from build123d import *

# Parameters (mm, degrees)
SKETCH1_W           = 152.4
SKETCH1_H           = 50.8
BOSS_EXTRUDE1_DEPTH = 6.35
SKETCH2_R           = 1.8288
CUT_EXTRUDE1_DEPTH  = 6.35
SKETCH5_W           = 8.89
SKETCH5_H           = 11.765011578
CUT_EXTRUDE2_DEPTH  = 161.769159045


with BuildPart() as part:
    # Sketch1 → Boss-Extrude1 (new body)
    with BuildSketch(Plane(origin=(0, 0, 0), x_dir=(1, 0, 0), z_dir=(0, 1, 0))):
        with Locations((-76.2, 25.4)):
            Rectangle(SKETCH1_W, SKETCH1_H)
    extrude(amount=BOSS_EXTRUDE1_DEPTH)

    # Sketch2 → Cut-Extrude1 (cut)
    with BuildSketch(Plane(origin=(0, 6.35, 0), x_dir=(1, 0, 0), z_dir=(0, 1, 0))):
        with Locations(Location((-149.225, 44.45, 0), (0, 0, 270))):
            Circle(SKETCH2_R)
        with Locations(Location((-149.225, 25.4, 0), (0, 0, 270))):
            Circle(SKETCH2_R)
        with Locations(Location((-149.225, 6.35, 0), (0, 0, 270))):
            Circle(SKETCH2_R)
        with Locations(Location((-3.175, 25.4, 0), (0, 0, 270))):
            Circle(SKETCH2_R)
        with Locations(Location((-3.175, 44.45, 0), (0, 0, 270))):
            Circle(SKETCH2_R)
        with Locations(Location((-3.175, 6.35, 0), (0, 0, 270))):
            Circle(SKETCH2_R)
    extrude(amount=-CUT_EXTRUDE1_DEPTH, mode=Mode.SUBTRACT)

    # Sketch5 → Cut-Extrude2 (cut, through all)
    with BuildSketch(Plane(origin=(0, 6.35, 0), x_dir=(1, 0, 0), z_dir=(0, 1, 0))):
        with Locations((-117.221, 44.917494211)):
            Rectangle(SKETCH5_W, SKETCH5_H)
    extrude(amount=-CUT_EXTRUDE2_DEPTH, mode=Mode.SUBTRACT)


solid = part.part
Could you check a few things on this model? Use its own coordinates, in mm. A direction names the side the tool comes from. Coordinates: 2 decimals unless noted, no trailing zeros. Order: outer loops, then holes, each group sorted by start corner. A loop starts at its lowest first (then second) coordinate and runs counter-clockwise, first axis right, second up.
Q1. Will these pins go through, and if not, where does the flat tip stop? pin 1 (3 mm diameter, centred on x = -3.175, z = -6.35, fed in from +Y); pin 2 (3 mm diameter, centred on x = -118.5, y = 4.5, fed in from -Z) (3 decimals).
Q2. Which directions (+Z, -Z, +X, -X, +Y, -Y) give clear straight access to the entire face, cutting with the end or side of a thin tool? Please do faces 1 (the flat face through (-57, 3, -50.8)), 2 (the flat face through (-121.666, 3, -45)).
Q3. Please list where these lines run through material, in increasing order: L1, parallel to X at y = 1.75, z = -44.45; L2, parallel to X at y = 2.5, z = -6.35; L3, parallel to X at y = 1.25, z = -40.
Q4. Suppose I cut it at B-B on z = -6.35. Please give me the cut outline in (x, y).
Q5. Suppose I cut it at D-D on x = -116. Please give me the cut outline in (y, z), and give its area (3 significant figures).
Q6. Suppose I cut it at C-C on y = 4. Please give me the cut outline in (x, z) (3 decimals).
Q7. Suppose I cut it at A-A on z = -41. Please give me the cut outline in (x, y), and give its area (3 significant figures).
Answer:
1. pin 1: passes through
1. pin 2: stops at z = -39.035
2. face 1: -Z, +X, -X, +Y, -Y
2. face 2: -Z, +Y, -Y
3. L1: x = -152.4 to -151.05, -147.4 to -121.67, -112.78 to -5, -1.35 to 0
3. L2: x = -152.4 to -151.05, -147.4 to -5, -1.35 to 0
3. L3: x = -152.4 to -121.67, -112.78 to 0
4. outline: (-152.4, 0) - (-151.05, 0) - (-151.05, 6.35) - (-152.4, 6.35) - close; (-147.4, 0) - (-5, 0) - (-5, 6.35) - (-147.4, 6.35) - close; (-1.35, 0) - (0, 0) - (0, 6.35) - (-1.35, 6.35) - close
5. outline: (0, -39.03) - (6.35, -39.03) - (6.35, 0) - (0, 0) - close
5. area: 248 mm2
6. outline: (-152.4, -50.8) - (-121.666, -50.8) - (-121.666, -39.035) - (-112.776, -39.035) - (-112.776, -50.8) - (0, -50.8) - (0, 0) - (-152.4, 0) - close; hole circle Ø3.658 at (-149.225, -44.45); hole circle Ø3.658 at (-149.225, -25.4); hole circle Ø3.658 at (-149.225, -6.35); hole circle Ø3.658 at (-3.175, -44.45); hole circle Ø3.658 at (-3.175, -25.4); hole circle Ø3.658 at (-3.175, -6.35)
7. outline: (-152.4, 0) - (-121.67, 0) - (-121.67, 6.35) - (-152.4, 6.35) - close; (-112.78, 0) - (0, 0) - (0, 6.35) - (-112.78, 6.35) - close
7. area: 911 mm2
